Work out the finished part from the listing and answer in its coordinate system (mm). A direction names the side the tool comes from. Give positions to 0.01 mm unless a question says otherwise; leave off trailing zeros. Loops run counter-clockwise (first coordinate to the right, second up) from the corner with the lowest first, then second, coordinate; pieces in that order, holes last. Notation, with made-up numbers: M 8,-35 L 46,-35 A16 cw 46,-27 Z; hole C -12,33 d6. An arc over 180 degrees is marked long. Write item = value, one per line. Start each with the question number.
1. Section B-B on z = 301.5 is taken. Determine the outline of the cut face in (x, y), plus the area to 3 significant figures.
2. The mould has two halves that part along X. Classify faces 5 (the face through (54.93, -98.6, 8.54)), 6 (the face through (0, 5, 530)), 7 (the face through (-5, 5, 261)), 8 (the face through (2.5, 5, 393)): released by +X, released by -X, zero draft, split by the parting line, or undercut.
3. Flat-ended cylindrical pins translate along their axes: pin 1 Ø5 at (x, y) = (19, -83) entering from -Z; pin 2 Ø5 at (y, z) = (7, 392) entering from +X; pin 3 Ø10 at (x, y) = (-25, -68) entering from +Z; pin 4 Ø3 at (y, z) = (3, 394.5) entering from -X. Find the tip coordinate at first contact, or state that the pin passes through.
4. Section C-C on x = 24 is taken. Determine the outline of the cut face in (y, z), plus the area to 3 significant figures.
5. For faces 1 (the face through (37, 0, 4)), 2 (the face through (-52.06, -98.6, 13.57)), 3 (the face through (-2.5, 5, 392)), 4 (the face through (-37, 0, 4)), determine the directions among +Z, -Z, +X, -X, +Y, -Y from which every point of the face is accessible in a straight line to the end or side of a thin tool.
6. Section A-A on y = -120 is taken. Determine the outline of the cut face in (x, z), plus the area to 3 significant figures.
7. Consider L1, parallel to Z at x = 0, y = 2; L2, parallel to Z at x = 42.5, y = -170; L3, parallel to Y at x = -0.5, z = 425. Determine where each line is inside the solid, lowest interval first. Write a range as [from, to].
```python
from build123d import *

# Parameters (mm, degrees)
F1_DEPTH = 200
F2_W     = 10
F2_H     = 530
F2_R     = 2.5
F3_DEPTH = 10
F4_R     = 5


with BuildPart() as f1:
    # F0 (on Front) → F1 (new body)
    with BuildSketch(Plane.XZ):
        Polygon((-60, 17.3205080757), (-50, 0), (0, 0), (50, 0), (60, 17.3205080757), (55.6698729811, 19.8205080757), (47.1132486541, 5), (0, 5), (-47.1132486541, 5), (-55.6698729811, 19.8205080757), align=None)
    extrude(amount=F1_DEPTH)

    # F2 (on Front) → F3 (join)
    with BuildSketch(Plane.XZ):
        with Locations((0, 265)):
            Rectangle(F2_W, F2_H)
        with Locations((0, 107.5)):
            Circle(F2_R, mode=Mode.SUBTRACT)
        with BuildLine():
            ThreePointArc((-2.5, 397.5), (0, 400), (2.5, 397.5))
            Line((2.5, 397.5), (2.5, 387.5))
            ThreePointArc((2.5, 387.5), (0, 385), (-2.5, 387.5))
            Line((-2.5, 387.5), (-2.5, 397.5))
        make_face(mode=Mode.SUBTRACT)
    extrude(amount=-F3_DEPTH)

    # F4
    f4_edges = [f1.edges().sort_by_distance(p)[0] for p in [
        (47.113249, -100, 5),
        (-47.113249, -100, 5),
        (5, 0, 2.5),
        (-5, 0, 2.5),
    ]]
    fillet(f4_edges, radius=F4_R)


solid = f1.part
```
Verdict:
q1.outline = M -5,0 L 5,0 L 5,10 L -5,10 Z
q1.area = 100 mm2
q2.face_5 = released by +X
q2.face_6 = zero draft
q2.face_7 = released by -X
q2.face_8 = undercut
q3.pin_1 = 0
q3.pin_2 = 5
q3.pin_3 = 5
q3.pin_4 = -5
q4.outline = M -200,0 L 0,0 L 0,5 L -200,5 Z
q4.area = 1,000 mm2
q5.face_1 = +Z, -Z, +X, +Y
q5.face_2 = +Z, +Y, -Y
q5.face_3 = +Y, -Y
q5.face_4 = +Z, -Z, -X, +Y
q6.outline = M -60,17.32 L -50,0 L 50,0 L 60,17.32 L 55.67,19.82 L 48.56,7.5 A5 cw 44.23,5 L -44.23,5 A5 cw -48.56,7.5 L -55.67,19.82 Z
q6.area = 674 mm2
q7.L1 = [0, 105], [110, 385], [400, 530]
q7.L2 = [0, 5]
q7.L3 = [0, 10]
